Here's how the part is built. I have some questions about the finished solid (model axes, mm). A direction names the side the tool comes from. Give positions to 0.01 mm unless a question says otherwise; leave off trailing zeros. Write each loop counter-clockwise with the first axis right and the second up, starting at its lowest first coordinate (ties: lowest second). Pieces come first, ordered by that corner, then holes. Notation, with made-up numbers: (-24.5, 69) -> (11.5, 69) arc R19 ccw to (11.5, 85) -> close; hole circle Ø11 at (-37.5, -23.5). An arc over 180 degrees is marked (long way). Return JSON: item names as keys, results as strings.
from build123d import *

# Parameters (mm, degrees)
F1_DEPTH = 203.2


with BuildPart() as f1:
    # F0 (on Front) → F1 (new body)
    with BuildSketch(Plane.XZ):
        with BuildLine():
            ThreePointArc((4, -6.928203), (6.928203, -4), (8, 0))
            ThreePointArc((8, 0), (-4, 6.928203), (-4, -6.928203))
            ThreePointArc((-4, -6.928203), (0, -8), (4, -6.928203))
        make_face()
        with BuildLine():
            ThreePointArc((4, -6.928203), (0, -8), (-4, -6.928203))
            Line((-4, -6.928203), (-7.678759, -13.3))
            Line((-7.678759, -13.3), (-9.25, -13.3))
            Line((-9.25, -13.3), (-9.25, -20))
            Line((-9.25, -20), (-20, -20))
            Line((-20, -20), (-20, -25))
            Line((-20, -25), (0, -25))
            Line((0, -25), (20, -25))
            Line((20, -25), (20, -20))
            Line((20, -20), (9.25, -20))
            Line((9.25, -20), (9.25, -13.3))
            Line((9.25, -13.3), (7.678759, -13.3))
            Line((7.678759, -13.3), (4, -6.928203))
        make_face()
    extrude(amount=F1_DEPTH)


solid = f1.part
1. If we mould it in two halves opening along Z, with no side actions, what happens to faces 1 (the face through (0, -203.2, -12)), 2 (the face through (0, -100, -25)), 3 (the face through (5.865, -100.178, -10.159)), 4 (the face through (-15, -100, -20))? For each: released by +Z, released by -Z, zero draft, split by the parting line, or undercut.
Taken from the geometry:
{"face 1": "zero draft", "face 2": "released by -Z", "face 3": "undercut", "face 4": "released by +Z"}
2. If I drill on line 1 (Z direction, x = -11.5, y = -189); line 2 (X direction, y = -15, z = -17); line 3 (Z direction, x = 4.5, y = -37), over which ranges is the centre line in solid material (lowest first)? Write a range as [from, to].
Taken from the geometry:
{"line 1": "z = [-25, -20]", "line 2": "x = [-9.25, 9.25]", "line 3": "z = [-25, -7.79], [-6.61, 6.61]"}
3. Suppose I cut it at C-C, the plane z = -11. List the corners of the cut face in (x, y) for me.
Taken from the geometry:
{"outline": "(-6.35, -203.2) -> (6.35, -203.2) -> (6.35, 0) -> (-6.35, 0) -> close"}
4. Suppose I cut it at A-A, the plane y = -128.5. List the corners of the cut face in (x, z) for me, and give its area (3 significant figures).
Taken from the geometry:
{"outline": "(-20, -25) -> (20, -25) -> (20, -20) -> (9.25, -20) -> (9.25, -13.3) -> (7.68, -13.3) -> (4, -6.93) arc R8 ccw (long way) to (-4, -6.93) -> (-7.68, -13.3) -> (-9.25, -13.3) -> (-9.25, -20) -> (-20, -20) -> close", "area": "594 mm²"}
5. Which directions (+Z, -Z, +X, -X, +Y, -Y) give clear straight access to the entire face, cutting with the end or side of a thin tool? Please do faces 5 (the face through (-9.25, -100, -17)), 6 (the face through (-5.814, -100.178, -10.069)), 7 (the face through (15, -100, -20)).
Taken from the geometry:
{"face 5": "+Z, -X, +Y, -Y", "face 6": "-X, +Y, -Y", "face 7": "+Z, +X, +Y, -Y"}
6. For pin 1 Ø3 at (y, z) = (-20.5, -6.5) entering from -X (3 decimals); pin 2 Ø3.5 at (y, z) = (-75.5, -16.5) entering from -X; pin 3 Ø8 at (y, z) = (-79.5, -0.5) entering from -X; pin 4 Ø12 at (x, z) = (15, -5) entering from -Y, each with a flat end and sliding along its axis, tell me the tip position at first contact or that it passes through.
Taken from the geometry:
{"pin 1": "stops at x = -6.245", "pin 2": "stops at x = -9.25", "pin 3": "stops at x = -8", "pin 4": "passes through"}
7. Suppose I cut it at B-B, the plane x = 12. List the corners of the cut face in (y, z) for me, and give its area (3 significant figures).
Taken from the geometry:
{"outline": "(-203.2, -25) -> (0, -25) -> (0, -20) -> (-203.2, -20) -> close", "area": "1,020 mm²"}
